Verification items for the finished model (mm, model axes). A direction names the side the tool comes from. Round coordinates to 2 decimals unless told otherwise and drop trailing zeros. Write each loop counter-clockwise with the first axis right and the second up, starting at its lowest first coordinate (ties: lowest second). Pieces come first, ordered by that corner, then holes. Notation, with made-up numbers: M 29.5,62 L 41.5,62 A26 ccw 41.5,93 Z; hole C -18,12.25 d6. An arc over 180 degrees is marked long. One line per question, with ' | ' between items. Start each with the question number.
Q1. Cross-section at A-A (y = -10). Record the boundary of the cut face in (x, z).
Q2. Tool access check on faces 1 (the face through (-1, -22, -10)), 2 (the face through (-4.51, -1.45, 12.35)), 3 (the face through (-4, -22, 14)), 4 (the face through (-4.51, -43.55, 12.35)), 5 (the face through (34.284, -40.453, -1.126)). Record the directions out of +Z, -Z, +X, -X, +Y, -Y that give a thin tool (end or side, any length) a straight path to the whole face; none if there is none.
Q3. Cross-section at B-B (z = -1.5). Record the boundary of the cut face in (x, y).
Q4. Release check for a two-part mould opening along Y. For faces 6 (the face through (4.295, -43.472, 12.246)), 7 (the face through (-1, 0, 3)), 8 (the face through (37.4, -7.6, 8)) record: released by +Y, released by -Y, zero draft, split by the parting line, or undercut.
Q5. Cross-section at C-C (x = -35). Record the boundary of the cut face in (y, z).
Q6. Gauge pin test, flat ends, axial feed: pin 1 (5.5 mm diameter, centred on x = -35.5, y = -32.5, fed in from -Z); pin 2 (5.5 mm diameter, centred on x = 35, y = -10, fed in from -Z). Record the tip position at first contact, or that the pin passes through.
Q7. Thickness scan on line 1 along Y through (x, z) = (-35, 14.25); line 2 along Y through (x, z) = (35, -1); line 3 along X through (y, z) = (-36, 2.5). Record the ranges inside material, lowest first. Write a range as from..to.
Q8. Cross-section at D-D (z = 16.75). State how many separate pieces and enclosed holes the cut face has, then the cut area to 3 significant figures.
from build123d import *

# Parameters (mm, degrees)
F1_DEPTH       = 45
F2_R           = 7.62
F3_R           = 5.08
F5_D           = 6
F5_CBORE_D     = 11
F5_CBORE_DEPTH = 18


with BuildPart() as f1:
    # F0 (on Front) → F1 (new body)
    with BuildSketch(Plane.XZ):
        Polygon((50, 20), (20, 20), (10, 20), (0, 10), (-10, 20), (-20, 20), (-50, 20), (-50, 0), (-50, -10), (50, -10), (50, 0), align=None)
    extrude(amount=F1_DEPTH)

    # F2
    f2_edges = [f1.edges().sort_by_distance(p)[0] for p in [
        (10, -22.5, 20),
        (-10, -22.5, 20),
    ]]
    fillet(f2_edges, radius=F2_R)

    # F3
    f3_edges = [f1.edges().sort_by_distance(p)[0] for p in [
        (-31.578154, -45, 20),
        (31.578154, -45, 20),
        (31.578154, 0, 20),
        (-31.578154, 0, 20),
    ]]
    fillet(f3_edges, radius=F3_R)

    # F5 (through all)
    with Locations(Plane(origin=(0, 0, -10), x_dir=(1, 0, 0), z_dir=(0, 0, -1))):
        with Locations((35, 10), (35, 35), (-35, 35), (-35, 10)):
            CounterBoreHole(F5_D / 2, F5_CBORE_D / 2, F5_CBORE_DEPTH)


solid = f1.part
Determined:
1) outline: M -50,-10 L -40.5,-10 L -40.5,8 L -38,8 L -38,20 L -50,20 Z; M -32,8 L -29.5,8 L -29.5,-10 L 29.5,-10 L 29.5,8 L 32,8 L 32,20 L 13.16,20 A7.62 ccw 7.77,17.77 L 0,10 L -7.77,17.77 A7.62 ccw -13.16,20 L -32,20 Z; M 38,8 L 40.5,8 L 40.5,-10 L 50,-10 L 50,20 L 38,20 Z
2) face 1: -Z, +X, -X, +Y, -Y | face 2: +Z, +Y | face 3: +Z, +Y, -Y | face 4: +Z, -Y | face 5: -Z
3) outline: M -50,-45 L 50,-45 L 50,0 L -50,0 Z; hole C -35,-35 d11; hole C -35,-10 d11; hole C 35,-35 d11; hole C 35,-10 d11
4) face 6: released by -Y | face 7: released by +Y | face 8: undercut
5) outline: M -45,-10 L -40.5,-10 L -40.5,8 L -38,8 L -38,20 L -39.92,20 A5.08 ccw -45,14.92 Z; M -32,8 L -29.5,8 L -29.5,-10 L -15.5,-10 L -15.5,8 L -13,8 L -13,20 L -32,20 Z; M -7,8 L -4.5,8 L -4.5,-10 L 0,-10 L 0,14.92 A5.08 ccw -5.08,20 L -7,20 Z
6) pin 1: stops at z = 8 | pin 2: passes through
7) line 1: y = -45..-38, -32..-13, -7..0 | line 2: y = -45..-40.5, -29.5..-15.5, -4.5..0 | line 3: x = -50..-40.41, -29.59..29.59, 40.41..50
8) separate pieces: 2 | enclosed holes: 4 | area: 3,700 mm²
